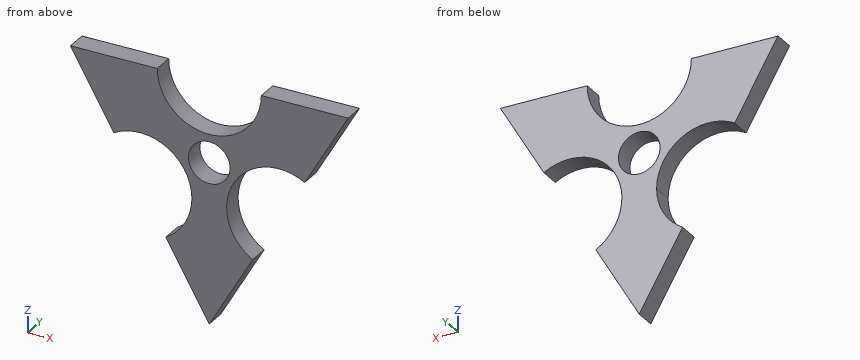
```python
from build123d import *

# Parameters (mm, degrees)
SKETCH1_R           = 3
BOSS_EXTRUDE1_DEPTH = 3


with BuildPart() as part:
    # Sketch1 → Boss-Extrude1 (new body)
    with BuildSketch(Plane(origin=(0, 0, 0), x_dir=(1, 0, 0), z_dir=(0, 1, 0))):
        with BuildLine():
            Line((6.555052507, 23.815698604), (0.305052507, 34.641016151))
            Line((0.305052507, 34.641016151), (-5.944947493, 23.815698604))
            ThreePointArc((-5.944947493, 23.815698604), (-3.199756965, 21.070508076), (-2.194947493, 17.320508076))
            ThreePointArc((-2.194947493, 17.320508076), (-5.944947493, 10.825317547), (-13.444947493, 10.825317547))
            Line((-13.444947493, 10.825317547), (-19.694947493, 0))
            Line((-19.694947493, 0), (-7.194947493, 0))
            ThreePointArc((-7.194947493, 0), (0.305052507, 7.5), (7.805052507, 0))
            Line((7.805052507, 0), (20.305052507, 0))
            Line((20.305052507, 0), (14.055052507, 10.825317547))
            ThreePointArc((14.055052507, 10.825317547), (3.809861978, 13.570508076), (6.555052507, 23.815698604))
        make_face()
        with Locations(Location((0.305052507, 11.551965164, 0), (0, 0, 270))):
            Circle(SKETCH1_R, mode=Mode.SUBTRACT)
    extrude(amount=BOSS_EXTRUDE1_DEPTH)


solid = part.part
```
Part model, mm, in its own coordinate system. Give positions to 0.01 mm unless a question says otherwise; leave off trailing zeros. Order: outer loops, then holes, each group sorted by start corner. A loop starts at its lowest first (then second) coordinate and runs counter-clockwise, first axis right, second up. Notation, with made-up numbers: M -7,12 L 8,12 A6 cw 8,16 Z; hole C 28.5,-9.75 d10. An arc over 180 degrees is marked long. Use a Markdown table: item, result. Add a question column.
(1) Saw through at B-B, the plane y = 2.2. Give the cut face in (x, z), and give its area (3 significant figures).
(2) Saw through at D-D, the plane x = 17. Give the cut face in (y, z).
(3) Saw through at A-A, the plane x = -0.5. Give the cut face in (y, z).
(4) Probe line 1 along Z through (x, y) = (-5, 2.4); line 2 along Z through (x, y) = (1, 0.75); line 3 along X through (y, z) = (0.7, -14). List the from-to ranges inside material, lowest first. Write a range as [from, to].
(5) Drop flat-ended pins along their axis: P1, Ø1.5, axis at x = -2.5, y = 1, coming from the -Z side; P2, Ø1.5, axis at y = 2, z = -28.5, coming from the -X side; P3, Ø1.5, axis at x = -0.5, y = 1.5, coming from the -Z side. Give the stop position or say it passes through.
(6) Saw through at C-C, the plane z = -7. Give the cut face in (x, y), and give its area (3 significant figures).
Answer key:
| question | item | result |
|---|---|---|
| 1 | outline | M -19.69,0 L -13.44,-10.83 A7.5 cw -5.94,-23.82 L 0.31,-34.64 L 6.56,-23.82 A7.5 cw 14.06,-10.83 L 20.31,0 L 7.81,0 A7.5 cw -7.19,0 Z; hole C 0.31,-11.55 d6 |
| 1 | area | 399 mm^2 |
| 2 | outline | M 0,-5.72 L 3,-5.72 L 3,0 L 0,0 Z |
| 3 | outline | M 0,-33.25 L 3,-33.25 L 3,-14.44 L 0,-14.44 Z; M 0,-8.66 L 3,-8.66 L 3,-7.46 L 0,-7.46 Z |
| 4 | line 1 | [-25.45, -23.17], [-11.47, -5.3] |
| 4 | line 2 | [-33.44, -14.47], [-8.63, -7.47] |
| 4 | line 3 | [-2.97, -1.43], [2.04, 3.58] |
| 5 | P1 | z = -31.08 |
| 5 | P2 | x = -3.67 |
| 5 | P3 | z = -34.55 |
| 6 | outline | M -15.65,0 L -2.39,0 L -2.39,3 L -15.65,3 Z; M 3,0 L 16.26,0 L 16.26,3 L 3,3 Z |
| 6 | area | 79.6 mm^2 |
